```python
from build123d import *

# Parameters (mm, degrees)
SKETCH1_R           = 3.875
BOSS_EXTRUDE1_DEPTH = 39.78
SKETCH2_OUTSIDE_W   = 18.002
SKETCH2_OUTSIDE_H   = 18.002
SKETCH2_OUTSIDE_R   = 2.39
CUT_EXTRUDE1_DEPTH  = 35
CHAMFER1_SIZE       = 0.5
CUT_EXTRUDE2_DEPTH  = 3.36


with BuildPart() as part:
    # Sketch1 → Boss-Extrude1 (new body)
    with BuildSketch(Plane(origin=(0, 0, 0), x_dir=(1, 0, 0), z_dir=(0, 1, 0))):
        Circle(SKETCH1_R)
    extrude(amount=BOSS_EXTRUDE1_DEPTH)

    # Sketch2 outside → Cut-Extrude1 (cut)
    with BuildSketch(Plane(origin=(0, 39.78, 0), x_dir=(1, 0, 0), z_dir=(0, 1, 0))):
        Rectangle(SKETCH2_OUTSIDE_W, SKETCH2_OUTSIDE_H)
        Circle(SKETCH2_OUTSIDE_R, mode=Mode.SUBTRACT)
    extrude(amount=-CUT_EXTRUDE1_DEPTH, mode=Mode.SUBTRACT)

    # Chamfer1
    chamfer1_edges = [part.edges().sort_by_distance(p)[0] for p in [
        (-2.39, 39.78, 0),
    ]]
    chamfer(chamfer1_edges, length=CHAMFER1_SIZE)

    # Sketch8 → Cut-Extrude2 (cut)
    with BuildSketch(Plane.XZ):
        Polygon((2.644264233, 0), (1.322132116, 2.29), (-1.322132116, 2.29), (-2.644264233, 0), (-1.322132116, -2.29), (1.322132116, -2.29), align=None)
    extrude(amount=-CUT_EXTRUDE2_DEPTH, mode=Mode.SUBTRACT)


solid = part.part
```
Can you work these out from the model? Positions are in its coordinate system, mm. A direction names the side the tool comes from. Coordinates: 2 decimals unless noted, no trailing zeros. Loops run counter-clockwise (first coordinate to the right, second up) from the corner with the lowest first, then second, coordinate; pieces in that order, holes last. Notation, with made-up numbers: (-35, 44.5) -> (-2, 44.5) arc R13 cw to (-2, 68.5) -> close; hole circle Ø8 at (39.5, 13.25). An arc over 180 degrees is marked (long way). Put each result on its own line as item: value. Start each with the question number.
Q1. For faces 1 (the face through (-1.974, 1.656, 1.161)), 2 (the face through (-0.504, 2.357, -3.842)), which set-ups out of +Z, -Z, +X, -X, +Y, -Y let a thin tool reach every point of the face, with its end or its side?
Q2. I want a section at C-C (y = 27). Write out the boundary of the cut face in (x, z).
Q3. Thinking about a two-plate mould opening in Z: for faces 3 (the face through (2.28, 22.27, -0.72)), 4 (the face through (-2, 4.78, 2)), 5 (the face through (-1.99, 1.66, -1.13)), which applies, pulls with the +Z half, pulls with the -Z half, needs draft (parallel to the pull), parting line crosses it, or undercut?
Q4. If I drill on line 1 (Y direction, x = 2.25, z = 2.75); line 2 (Y direction, x = -0.25, z = 0); line 3 (Z direction, x = 0, y = 36), over which ranges is the centre line in solid material (lowest first)? Write a range as [from, to].
Q5. I want a section at A-A (y = 3). Write out the boundary of the cut face in (x, z) (3 decimals).
Q6. I want a section at B-B (x = 0). Write out the boundary of the cut face in (y, z) (3 decimals).
Q7. I'm going to push flat-ended pins straight in: P1, Ø2, axis at x = 0.5, y = 1.5, coming from the +Z side (3 decimals); P2, Ø1, axis at x = 0.5, y = 18, coming from the -Z side; P3, Ø3, axis at x = 2.5, z = -2.5, coming from the +Y side; P4, Ø4, axis at y = 19, z = -2.5, coming from the -X side. Where does each tip first touch, or does it pass through?
Q8. I want a section at D-D (z = -2.75). Write out the boundary of the cut face in (x, y), plus the area to 3 significant figures.
Taken from the geometry:
1. face 1: -Y
1. face 2: +Y, -Y
2. outline: circle Ø4.78 at (0, 0)
3. face 3: parting line crosses it
3. face 4: needs draft
3. face 5: undercut
4. line 1: y = [0, 4.78]
4. line 2: y = [3.36, 39.78]
4. line 3: z = [-2.39, 2.39]
5. outline: circle Ø7.75 at (0, 0); hole (-2.644, 0) -> (-1.322, -2.29) -> (1.322, -2.29) -> (2.644, 0) -> (1.322, 2.29) -> (-1.322, 2.29) -> close
6. outline: (0, -3.875) -> (4.78, -3.875) -> (4.78, -2.39) -> (39.28, -2.39) -> (39.78, -1.89) -> (39.78, 1.89) -> (39.28, 2.39) -> (4.78, 2.39) -> (4.78, 3.875) -> (0, 3.875) -> (0, 2.29) -> (3.36, 2.29) -> (3.36, -2.29) -> (0, -2.29) -> close
7. P1: stops at z = 3.875
7. P2: stops at z = -2.39
7. P3: stops at y = 39.63
7. P4: stops at x = -2.34
8. outline: (-2.73, 0) -> (2.73, 0) -> (2.73, 4.78) -> (-2.73, 4.78) -> close
8. area: 26.1 mm2
